```python
from build123d import *

# Parameters (mm, degrees)
SKETCH1_R         = 49
SKETCH1_R_2       = 38.7985
EXTRUDE1_DEPTH    = 35.306
SKETCH2_OUTSIDE_W = 128.604
SKETCH2_OUTSIDE_H = 128.604
SKETCH2_OUTSIDE_R = 46.228
EXTRUDE2_DEPTH    = 22.606
SKETCH3_R         = 41.1607
EXTRUDE3_DEPTH    = 23.5712
CHAMFER1_SIZE     = 3.175
CHAMFER1_SIZE2    = 12.7


with BuildPart() as part:
    # Sketch1 → Extrude1 (new body)
    with BuildSketch(Plane.XY):
        Circle(SKETCH1_R)
        Circle(SKETCH1_R_2, mode=Mode.SUBTRACT)
    extrude(amount=EXTRUDE1_DEPTH)

    # Sketch2 outside → Extrude2 (cut)
    with BuildSketch(Plane.XY.offset(35.306)):
        Rectangle(SKETCH2_OUTSIDE_W, SKETCH2_OUTSIDE_H)
        Circle(SKETCH2_OUTSIDE_R, mode=Mode.SUBTRACT)
    extrude(amount=-EXTRUDE2_DEPTH, mode=Mode.SUBTRACT)

    # Sketch3 → Extrude3 (cut)
    with BuildSketch(Plane(origin=(0, 0, 0), x_dir=(-1, 0, 0), z_dir=(0, 0, -1))):
        Circle(SKETCH3_R)
    extrude(amount=-EXTRUDE3_DEPTH, mode=Mode.SUBTRACT)

    # Chamfer1
    chamfer1_edges = [part.edges().sort_by_distance(p)[0] for p in [
        (41.1607, 0, 0),
    ]]
    chamfer1_side = [part.faces().sort_by_distance(p)[0] for p in [
        (-47.614070709, 0, 0),
    ]]
    chamfer(chamfer1_edges, length=CHAMFER1_SIZE, length2=CHAMFER1_SIZE2, reference=chamfer1_side[0])


solid = part.part
```
The listing builds one solid part. Answer for the finished solid, in the listing's coordinates (mm). A direction names the side the tool comes from. Coordinates: 2 decimals unless noted, no trailing zeros. Loops run counter-clockwise (first coordinate to the right, second up) from the corner with the lowest first, then second, coordinate; pieces in that order, holes last. Notation, with made-up numbers: M 4,15.5 L 55,15.5 A21 cw 55,22.5 Z; hole C 68,11 d1. An arc over 180 degrees is marked long. Answer as CSV lines item,"result". Start each with the question number.
(1) The mould has two halves that part along Y. Classify faces 3 (the cylindrical face through (24.85, 38.98, 24.16)), 4 (the flat face through (-37, -25, 0)), 5 (the cylindrical face through (30.337, 27.818, 18.06)), 6 (the flat face through (28, 28, 23.571)): pulls with the +Y half, pulls with the -Y half, needs draft (parallel to the pull), parting line crosses it, or undercut.
(2) Find the intervals of material crossed by L1, parallel to Y at x = 0, z = 21; L2, parallel to Y at x = 0, z = 27; L3, parallel to X at y = 11, z = 24, in increasing order. Write a range as [from, to].
(3) The part is cut by section C-C (z = 27.5). Give the vertices of the cut face in (x, y), and give its area (3 significant figures).
(4) For faces 1 (the conical face through (5.378, 40.963, 12.083)), 2 (the flat face through (36.1, 29.3, 12.7)), determine the directions among +Z, -Z, +X, -X, +Y, -Y from which every point of the face is accessible in a straight line to the end or side of a thin tool.
(5) The part is cut by section A-A (y = 0). Give the vertices of the cut face in (x, z).
(6) Given pin 1 (1 mm diameter, centred on x = -30, z = 10.5, fed in from -Y); pin 2 (2 mm diameter, centred on x = 21, z = 13.5, fed in from +Y); pin 3 (6 mm diameter, centred on x = -38.5, z = 4, fed in from +Y) (3 decimals), each flat-ended and moving along its own axis, determine where each tip first touches the part or whether it passes through.
Determined:
1,face 3,"parting line crosses it"
1,face 4,"needs draft"
1,face 5,"undercut"
1,face 6,"undercut"
2,L1,"[-46.23, -41.16], [41.16, 46.23]"
2,L2,"[-46.23, -38.8], [38.8, 46.23]"
2,L3,"[-44.9, -37.21], [37.21, 44.9]"
3,outline,"C 0,0 d92.46; hole C 0,0 d77.6"
3,area,"1,980 mm2"
4,face 1,"-Z"
4,face 2,"+Z"
5,outline,"M -49,0 L -44.34,0 L -41.16,12.7 L -41.16,23.57 L -38.8,23.57 L -38.8,35.31 L -46.23,35.31 L -46.23,12.7 L -49,12.7 Z; M 38.8,23.57 L 41.16,23.57 L 41.16,12.7 L 44.34,0 L 49,0 L 49,12.7 L 46.23,12.7 L 46.23,35.31 L 38.8,35.31 Z"
6,pin 1,"y = -39.12"
6,pin 2,"y = 44.55"
6,pin 3,"y = 33.775"
